Can you work these out from the model? Positions are in its coordinate system, mm. Face numbers are marked on the shaded views. Coordinates: 2 decimals unless noted, no trailing zeros. Order: outer loops, then holes, each group sorted by start corner. A loop starts at its lowest first (then second) coordinate and runs counter-clockwise, first axis right, second up. Notation, with made-up numbers: (-33, 88.25) -> (-17, 88.25) arc R19 ccw to (-17, 100.25) -> close; hole circle Ø3 at (8, -9.75). An arc over 180 degrees is marked (long way). Answer as a JSON object with one key per item and string values. Group by question number.
(1) I want a section at B-B, the plane x = 11. List the corners of the cut face in (y, z) for me.
(2) I want a section at A-A, the plane y = -5.5. List the corners of the cut face in (x, z) for me, plus the area to 3 significant figures.
(3) For pin 1 (8 mm diameter, centred on x = -14, y = 1.5, fed in from -Z), with a flat end and sliding along its axis, tell me the tip position at first contact or that it passes through.
(4) If we mould it in two halves opening along X, with no side actions, what happens to the marked faces 1 and 2? For each: pulls with the +X half, pulls with the -X half, needs draft (parallel to the pull), parting line crosses it, or undercut.
(5) I need wall thicknesses on line 1 (Z direction, x = -2, y = 4); line 2 (X direction, y = 0.25, z = 2.35); line 3 (X direction, y = -13.5, z = 2.3). Which ranges of each line are inside material? Lowest first, please.
from build123d import *

# Parameters (mm, degrees)
F1_DEPTH = 15
F2_R     = 0.5


with BuildPart() as f1:
    # F0 (on Front) → F1 (new body, symmetric)
    with BuildSketch(Plane.XZ):
        Polygon((-24.5, 1.5), (-24.5, 0), (24.5, 0), (24.5, 1.5), (22.5, 1.5), (-22.5, 1.5), align=None)
        Polygon((-24.5, 3.5), (-24.5, 1.5), (-22.5, 1.5), align=None)
        Polygon((22.5, 1.5), (24.5, 1.5), (24.5, 3.5), align=None)
    extrude(amount=F1_DEPTH, both=True)

    # F2
    f2_edges = [f1.edges().sort_by_distance(p)[0] for p in [
        (-24.5, 0, 3.5),
        (24.5, 0, 3.5),
    ]]
    fillet(f2_edges, radius=F2_R)


solid = f1.part
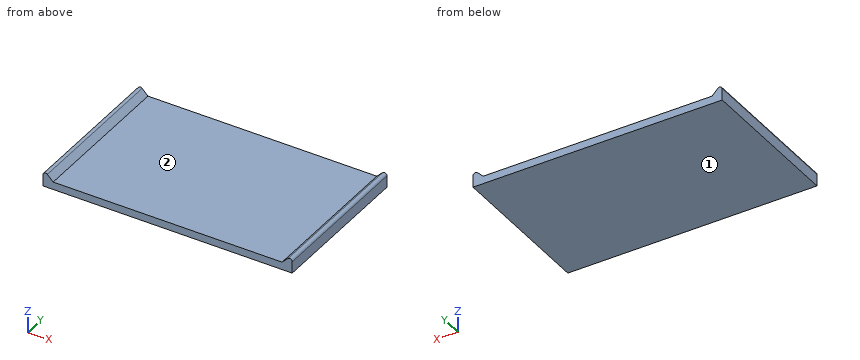
Computed values:
{
 "1": {"outline": "(-15, 0) -> (15, 0) -> (15, 1.5) -> (-15, 1.5) -> close"},
 "2": {"outline": "(-24.5, 0) -> (24.5, 0) -> (24.5, 2.29) arc R0.5 ccw to (23.65, 2.65) -> (22.5, 1.5) -> (-22.5, 1.5) -> (-23.65, 2.65) arc R0.5 ccw to (-24.5, 2.29) -> close", "area": "76.9 mm2"},
 "3": {"pin 1": "stops at z = 0"},
 "4": {"face 1": "needs draft", "face 2": "undercut"},
 "5": {"line 1": "z = 0 to 1.5", "line 2": "x = -24.5 to -23.35, 23.35 to 24.5", "line 3": "x = -24.5 to -23.3, 23.3 to 24.5"}
}
